Autodesk Inventor part; units mm, degrees
ref_plane "YZ Plane" through (0, 0, 0) normal (1, 0, 0) x (0, 1, 0)
ref_plane "XZ Plane" through (0, 0, 0) normal (0, 1, 0) x (-1, 0, 0)
ref_plane "XY Plane" through (0, 0, 0) normal (0, 0, 1) x (1, 0, 0)
sketch "Sketch1" plane through (0, 0, 0) normal (0, 1, 0) x (-1, 0, 0)
  circle A0 centre (0, 0) radius 12.5
  dimension "d0" = 25
extrude "Extrusion1" add sketch "Sketch1" along normal blind 29.3
hole "ReliefTop" at (0, 29.3, 0) direction (0, -1, 0) diameter 13.97 depth 0.254 countersink diameter 14.478 countersink angle 90
hole "ReliefBottom" at (0, 0, 0) direction (0, 1, 0) diameter 13.97 depth 0.254 countersink diameter 14.478 countersink angle 90
hole "MountBottomM6" at (0, 0.254, 0) direction (0, 1, 0) diameter 4.917 depth 7.366 tip angle 118 countersink diameter 5.508 countersink angle 90
hole "MountTopM4" at (0, 29.046, 0) direction (0, -1, 0) diameter 3.242 depth 14.478 tip angle 118 countersink diameter 3.808 countersink angle 90
sketch "Sketch2" plane through (0, 0, 0) normal (0, 0, 1) x (1, 0, 0)
  circle A0 centre (0, 20) radius 3
  line L0 (-12.5, 0) -> (12.5, 0)
  line L1 (0, -4.6) -> (0, 27.6)
  point P0 (0, 0)
  dimension "d49" = 6
  dimension "d50" = 20
extrude "Extrusion2" cut sketch "Sketch2" along normal through all both and the other way through all
chamfer "Chamfer1" distance 0.313 angle 45 2 edges at (-3, 19.9998, 12.1347) (-3, 19.9998, -12.1347)
extrude "Extrusion3" add sketch "Sketch2" along normal mid plane 14.84
equation "\"d1\" = height"
equation "\"d5\" = reliefMinor"
equation "\"d7\" = reliefMajor"
equation "\"d10\" = reliefDepth"
equation "\"d14\" = reliefMinor"
equation "\"d16\" = reliefMajor"
equation "\"d19\" = reliefDepth"
equation "\"d25\" = chamferM6"
equation "\"d28\" = depthM6"
equation "\"d40\" = chamferM4"
equation "\"d43\" = depthM4"
equation "\"reliefDepth\" = 0.254"
equation "\"reliefMinor\" = 13.97"
equation "\"reliefMajor\" = 14.478"
equation "\"chamferM6\" = 5.508"
equation "\"chamferM4\" = 3.808"
equation "\"depthM6\" = 7.366"
equation "\"depthM4\" = 14.478"
equation "\"height\" = 29.3"
properties part number "PLS-P642H0293A00_M" material "Stainless Steel"
Check sheet for the modelled part. Datum: model origin and axes. Units: mm. A direction names the side the tool comes from. Round coordinates to 2 decimals unless told otherwise and drop trailing zeros. Loops run counter-clockwise (first coordinate to the right, second up) from the corner with the lowest first, then second, coordinate; pieces in that order, holes last. Notation, with made-up numbers: (1, 3.25) -> (27, 3.25) arc R13 ccw to (27, 22.25) -> close; hole circle Ø1 at (48, -17.5). An arc over 180 degrees is marked (long way). Answer in a Markdown table with one row per item.
Q1. Set-up check for faces 1 (the face through (0, 20, 7.42)), 2 (the face through (-3, 20, -10)), 3 (the face through (-1.607, 25.6, -0.211)), 4 (the face through (-0.27, 13.76, -0.06)): record each of +Z, -Z, +X, -X, +Y, -Y from which the full face is reachable in a straight line by a thin tool's end or side.
Data:
| item | result |
|---|---|
| face 1 | +Z |
| face 2 | -Z |
| face 3 | +Y |
| face 4 | none |
Q2. Sectioned sample at C-C on x = 10.5. Enter the section's corners in (y, z), then the cut area to 3 significant figures.
Data:
| item | result |
|---|---|
| outline | (0, -6.78) -> (29.3, -6.78) -> (29.3, 6.78) -> (0, 6.78) -> close |
| area | 397 mm^2 |
Q3. Release check for a two-part mould opening along Z. For faces 5 (the face through (-0.738, 4.134, -2.345)), 6 (the face through (-5.4, 0, -5.4)), 7 (the face through (-5.77, 14.44, 11.09)) record: released by +Z, released by -Z, zero draft, split by the parting line, or undercut.
Data:
| item | result |
|---|---|
| face 5 | undercut |
| face 6 | zero draft |
| face 7 | split by the parting line |
Q4. Thickness scan on L1, parallel to Z at x = 0, y = 25; L2, parallel to Y at x = 0, z = -9.1; L3, parallel to Y at x = -1.75, z = 2.5. Record the ranges inside material, lowest first.
Data:
| item | result |
|---|---|
| L1 | z = -12.5 to -1.62, 1.62 to 12.5 |
| L2 | y = 0 to 17, 23 to 29.3 |
| L3 | y = 0.25 to 29.05 |
Q5. Sectioned sample at A-A on y = 4.75. Enter the section's corners in (x, z), then the cut area to 3 significant figures.
Data:
| item | result |
|---|---|
| outline | circle Ø25 at (0, 0); hole circle Ø4.92 at (0, 0) |
| area | 472 mm^2 |
Q6. Go/stop test with flat-tipped pins: P1, Ø4.5, axis at x = 0, z = 0, coming from the -Y side; P2, Ø2, axis at x = -2, y = 7.5, coming from the +Z side; P3, Ø4, axis at x = -1.5, z = -0.5, coming from the +Y side. Record where each tip stops, or that it passes through.
Data:
| item | result |
|---|---|
| P1 | stops at y = 7.75 |
| P2 | stops at z = 12.46 |
| P3 | stops at y = 29.05 |
Q7. Sectioned sample at B-B on z = -10.25. Enter the section's corners in (x, y).
Data:
| item | result |
|---|---|
| outline | (-7.15, 0) -> (7.15, 0) -> (7.15, 29.3) -> (-7.15, 29.3) -> close; hole circle Ø6 at (0, 20) |
Q8. Sectioned sample at D-D on y = 27.5. Enter the section's corners in (x, z), then the cut area to 3 significant figures.
Data:
| item | result |
|---|---|
| outline | circle Ø25 at (0, 0); hole circle Ø3.24 at (0, 0) |
| area | 483 mm^2 |
